The listing builds one solid part. Answer for the finished solid, in the listing's coordinates (mm). Face numbers are marked on the shaded views. A direction names the side the tool comes from. Coordinates: 2 decimals unless noted, no trailing zeros. Order: outer loops, then holes, each group sorted by start corner. A loop starts at its lowest first (then second) coordinate and runs counter-clockwise, first axis right, second up. Notation, with made-up numbers: (-24.75, 14) -> (-5.75, 14) arc R27 cw to (-5.75, 52) -> close; hole circle Ø6 at (5, 4). An arc over 180 degrees is marked (long way). Answer in a Markdown table with one row per item. Add a question column.
```python
from build123d import *

# Parameters (mm, degrees)
SKETCH1_W             = 100
SKETCH1_H             = 100
BOSS_EXTRUDE1_DEPTH   = 6
SKETCH2_W             = 15
SKETCH2_H             = 78.4
CUT_EXTRUDE1_DEPTH    = 1
M3_TAPPED_HOLE1_D     = 2.5
M3_TAPPED_HOLE1_DEPTH = 4
M3_TAPPED_HOLE1_TIP   = 0.751075774
SKETCH11_R            = 2
CUT_EXTRUDE3_DEPTH    = 1
FILLET2_R             = 3


with BuildPart() as part:
    # Sketch1 → Boss-Extrude1 (new body)
    with BuildSketch(Plane(origin=(0, 0, 0), x_dir=(1, 0, 0), z_dir=(0, 1, 0))):
        Rectangle(SKETCH1_W, SKETCH1_H)
    extrude(amount=BOSS_EXTRUDE1_DEPTH)

    # Sketch2 → Cut-Extrude1 (cut)
    with BuildSketch(Plane(origin=(0, 6, 0), x_dir=(1, 0, 0), z_dir=(0, 1, 0))):
        with Locations((-22.6, 0)):
            Rectangle(SKETCH2_W, SKETCH2_H)
        Rectangle(SKETCH2_W, SKETCH2_H)
        with Locations((22.6, 0)):
            Rectangle(SKETCH2_W, SKETCH2_H)
    extrude(amount=-CUT_EXTRUDE1_DEPTH, mode=Mode.SUBTRACT)

    # M3 Tapped Hole1
    with Locations(Plane(origin=(0, 6, 0), x_dir=(1, 0, 0), z_dir=(0, 1, 0))):
        with Locations((11.3, 19.6), (-33.9, 19.6), (33.9, 19.6), (-37.5, 37.5), (37.5, 37.5), (37.5, -37.5), (-37.5, -37.5), (-33.9, -19.6), (-11.3, -19.6), (11.3, -19.6), (33.9, -19.6), (-11.3, 19.6)):
            Hole(M3_TAPPED_HOLE1_D / 2, depth=M3_TAPPED_HOLE1_DEPTH)
            with Locations((0, 0, -(M3_TAPPED_HOLE1_DEPTH + M3_TAPPED_HOLE1_TIP / 2))):  # 118° drill point
                Cone(0, M3_TAPPED_HOLE1_D / 2, M3_TAPPED_HOLE1_TIP, mode=Mode.SUBTRACT)

    # Sketch11 → Cut-Extrude3 (cut)
    with BuildSketch(Plane(origin=(0, 6, 0), x_dir=(1, 0, 0), z_dir=(0, 1, 0))):
        with Locations((-30.1, 39.2)):
            Circle(SKETCH11_R)
        with Locations((-30.1, -39.2)):
            Circle(SKETCH11_R)
        with Locations((-15.1, -39.2)):
            Circle(SKETCH11_R)
        with Locations((-7.5, -39.2)):
            Circle(SKETCH11_R)
        with Locations((7.5, -39.2)):
            Circle(SKETCH11_R)
        with Locations((15.1, -39.2)):
            Circle(SKETCH11_R)
        with Locations((30.1, -39.2)):
            Circle(SKETCH11_R)
        with Locations((30.1, 39.2)):
            Circle(SKETCH11_R)
        with Locations((7.5, 39.2)):
            Circle(SKETCH11_R)
        with Locations((15.1, 39.2)):
            Circle(SKETCH11_R)
        with Locations((-7.5, 39.2)):
            Circle(SKETCH11_R)
        with Locations((-15.1, 39.2)):
            Circle(SKETCH11_R)
    extrude(amount=-CUT_EXTRUDE3_DEPTH, mode=Mode.SUBTRACT)

    # Fillet2
    fillet2_edges = [part.edges().sort_by_distance(p)[0] for p in [
        (50, 3, 50),
        (-50, 3, 50),
        (-50, 3, -50),
        (50, 3, -50),
    ]]
    fillet(fillet2_edges, radius=FILLET2_R)


solid = part.part
```
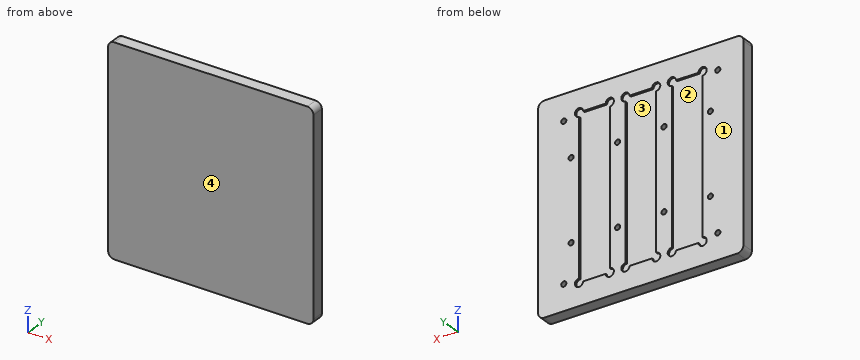
Q1. Straight lines are drawn through the part: line 1 (X direction, y = 3.95, z = -19.5); line 2 (Z direction, x = 33.9, y = 5); line 3 (X direction, y = 2.95, z = 37.5). For each, find the intervals that lie inside material, in ascending order.
Q2. A cutting plane is placed at A-A (x = 0). Determine the outline of the cut face in (y, z).
Q3. Determine the mould class of the marked faces 3 and 4 for opening direction X: +X half, -X half, draft (parallel to the pull), parting line (faces both ways), or undercut.
Q4. For the marked faces 1 and 2, determine the directions among +Z, -Z, +X, -X, +Y, -Y from which every point of the face is accessible in a straight line to the end or side of a thin tool.
Q5. Given pin 1 (2.5 mm diameter, centred on x = 7.5, z = -39.2, fed in from +Y); pin 2 (1.5 mm diameter, centred on x = -37.5, z = 37.5, fed in from +Y), each flat-ended and moving along its own axis, determine where each tip first touches the part or whether it passes through.
Q6. A cutting plane is placed at B-B (z = 27). Determine the outline of the cut face in (x, y).
Returned:
| question | item | result |
|---|---|---|
| 1 | line 1 | x = -50 to -35.15, -32.65 to -12.55, -10.05 to 10.05, 12.55 to 32.65, 35.15 to 50 |
| 1 | line 2 | z = -50 to -20.85, -18.35 to 18.35, 20.85 to 50 |
| 1 | line 3 | x = -50 to -38.75, -36.25 to 36.25, 38.75 to 50 |
| 2 | outline | (0, -50) -> (6, -50) -> (6, -39.2) -> (5, -39.2) -> (5, 39.2) -> (6, 39.2) -> (6, 50) -> (0, 50) -> close |
| 3 | face 3 | undercut |
| 3 | face 4 | draft |
| 4 | face 1 | +Z, -Z, +X, -X, +Y |
| 4 | face 2 | +Y |
| 5 | pin 1 | stops at y = 5 |
| 5 | pin 2 | stops at y = 1.7 |
| 6 | outline | (-50, 0) -> (50, 0) -> (50, 6) -> (30.1, 6) -> (30.1, 5) -> (15.1, 5) -> (15.1, 6) -> (7.5, 6) -> (7.5, 5) -> (-7.5, 5) -> (-7.5, 6) -> (-15.1, 6) -> (-15.1, 5) -> (-30.1, 5) -> (-30.1, 6) -> (-50, 6) -> close |
